Input: dimensioned drawing with shaded views. Units: mm. Origin: part minimum x, y, z. Round coordinates to 2 decimals unless told otherwise and drop trailing zeros. Loops run counter-clockwise (first coordinate to the right, second up) from the corner with the lowest first, then second, coordinate; pieces in that order, holes last. Notation, with made-up numbers: M -28.5,64 L -14.5,64 A7 ccw -14.5,69 Z; hole C 44,22.5 d4. An arc over 180 degrees is marked long. Use one line per item in the form item = value. Start each with the question number.
Q1. Mould query, pull axis X, two halves, no side actions, for the marked faces 1 and 2. Classes: pulls with the +X half, pulls with the -X half, needs draft (parallel to the pull), parting line crosses it, or undercut.
Q2. Section query B-B, the plane y = 60. Output: boundary loops of the cut face in (x, z).
Q3. Section query A-A, the plane x = 58. Output: boundary loops of the cut face in (y, z), and give its area (3 significant figures).
Q4. Ray query, line 1 along X through (y, z) = (18.5, 1.35); line 2 along Y through (x, z) = (32, 0.85); line 3 along X through (y, z) = (38, 0.95). Return the intervals inside material, ascending.
Q5. Section query C-C, the plane x = 32. Output: boundary loops of the cut face in (y, z).
Q6. First-contact query: P1, Ø2.5, axis at x = 98, y = 60, coming from the -Z side. Flat tip, straight axial feed; report the tip coordinate or a pass-through.
Q7. Section query D-D, the plane z = 3.5. Output: boundary loops of the cut face in (x, y), and give its area (3 significant figures).
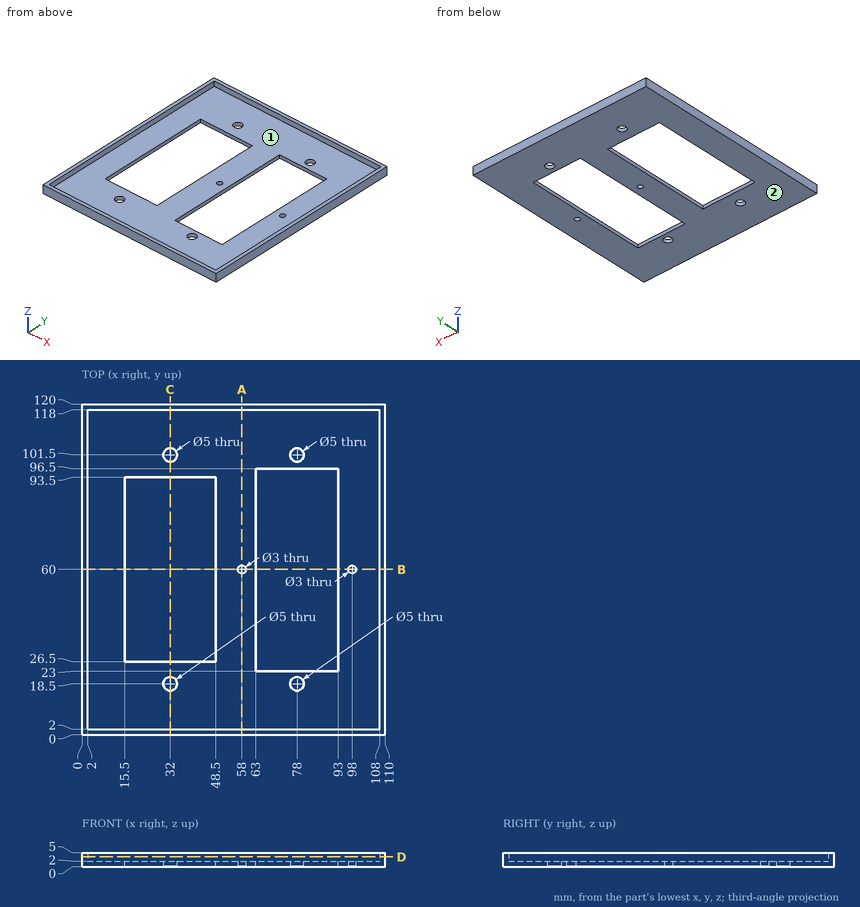
Results found:
q1.face_1 = undercut
q1.face_2 = needs draft
q2.outline = M 0,0 L 15.5,0 L 15.5,2 L 2,2 L 2,5 L 0,5 Z; M 48.5,0 L 56.5,0 L 56.5,2 L 48.5,2 Z; M 59.5,0 L 63,0 L 63,2 L 59.5,2 Z; M 93,0 L 96.5,0 L 96.5,2 L 93,2 Z; M 99.5,0 L 110,0 L 110,5 L 108,5 L 108,2 L 99.5,2 Z
q3.outline = M 0,0 L 58.5,0 L 58.5,2 L 2,2 L 2,5 L 0,5 Z; M 61.5,0 L 120,0 L 120,5 L 118,5 L 118,2 L 61.5,2 Z
q3.area = 246 mm²
q4.line_1 = 0 to 29.5, 34.5 to 75.5, 80.5 to 110
q4.line_2 = 0 to 16, 21 to 26.5, 93.5 to 99, 104 to 120
q4.line_3 = 0 to 15.5, 48.5 to 63, 93 to 110
q5.outline = M 0,0 L 16,0 L 16,2 L 2,2 L 2,5 L 0,5 Z; M 21,0 L 26.5,0 L 26.5,2 L 21,2 Z; M 93.5,0 L 99,0 L 99,2 L 93.5,2 Z; M 104,0 L 120,0 L 120,5 L 118,5 L 118,2 L 104,2 Z
q6.P1 = through
q7.outline = M 0,0 L 110,0 L 110,120 L 0,120 Z; hole M 2,2 L 108,2 L 108,118 L 2,118 Z
q7.area = 904 mm²
